from build123d import *

# Parameters (mm, degrees)
SKETCH2_W               = 70.5
SKETCH2_H               = 90
BOSS_EXTRUDE1_DEPTH     = 55.25
CUT_EXTRUDE1_DEPTH      = 91
SKETCH4_R               = 25
CUT_EXTRUDE2_DEPTH      = 45
SKETCH6_W               = 16.5
SKETCH6_H               = 50
CUT_EXTRUDE3_DEPTH      = 35.414718703
CUT_EXTRUDE3_DEPTH_BACK = 11
SKETCH7_W               = 25
SKETCH7_H               = 15
CUT_EXTRUDE4_DEPTH      = 15


with BuildPart() as part:
    # Sketch2 → Boss-Extrude1 (new body)
    with BuildSketch(Plane.XY):
        Rectangle(SKETCH2_W, SKETCH2_H)
    extrude(amount=BOSS_EXTRUDE1_DEPTH)

    # Sketch3 → Cut-Extrude1 (cut, through all)
    with BuildSketch(Plane.XZ.offset(45)):
        Polygon((28.75, 20.835281297), (35.25, 11), (35.25, 55.25), (8.75, 55.25), (8.75, 20.835281297), align=None)
    extrude(amount=-CUT_EXTRUDE1_DEPTH, mode=Mode.SUBTRACT)

    # Sketch4 → Cut-Extrude2 (cut, through all)
    with BuildSketch(Plane(origin=(8.75, 0, 0), x_dir=(0, 0, -1), z_dir=(1, 0, 0))):
        with Locations((-55.327535333, 0)):
            Circle(SKETCH4_R)
    extrude(amount=-CUT_EXTRUDE2_DEPTH, mode=Mode.SUBTRACT)

    # Sketch6 → Cut-Extrude3 (cut, two sides)
    with BuildSketch(Plane.XY.offset(20.835281297)) as cut_extrude3_sk:
        with Locations((27, 0)):
            Rectangle(SKETCH6_W, SKETCH6_H)
    extrude(amount=CUT_EXTRUDE3_DEPTH, mode=Mode.SUBTRACT)
    extrude(cut_extrude3_sk.sketch, amount=-CUT_EXTRUDE3_DEPTH_BACK, mode=Mode.SUBTRACT)

    # Sketch7 → Cut-Extrude4 (cut)
    with BuildSketch(Plane.XY.offset(55.25)):
        with Locations((-13.733691731, 26)):
            Rectangle(SKETCH7_W, SKETCH7_H)
        Polygon((-25.955312552, -17.750715844), (-0.958260941, -17.366774787), (-0.727896306, -32.365005754), (-25.724947918, -32.748946811), align=None)
    extrude(amount=-CUT_EXTRUDE4_DEPTH, mode=Mode.SUBTRACT)


solid = part.part
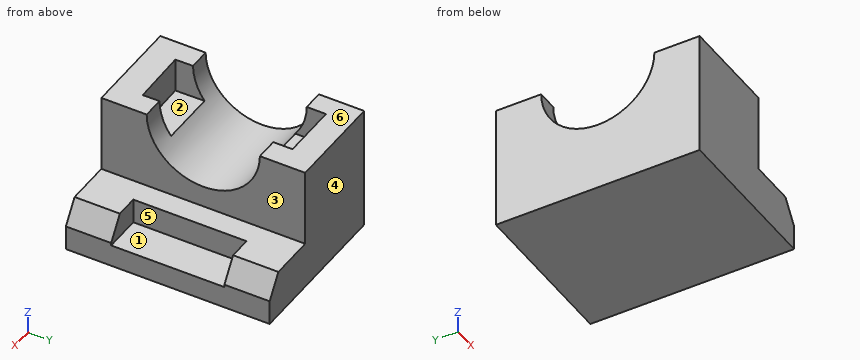
The listing builds one solid part. Answer for the finished solid, in the listing's coordinates (mm). Face numbers are marked on the shaded views. A direction names the side the tool comes from. Round coordinates to 2 decimals unless told otherwise and drop trailing zeros. Order: outer loops, then holes, each group sorted by start corner. A loop starts at its lowest first (then second) coordinate and runs counter-clockwise, first axis right, second up. Notation, with made-up numbers: (65.5, 81) -> (91.5, 81) arc R20 ccw to (91.5, 109) -> close; hole circle Ø5 at (68.25, 22). An arc over 180 degrees is marked (long way). Put each result on its own line as item: value.
Q1. Determine the mould class of the marked faces 4, 5 and 6 for opening direction Y: pulls with the +Y half, pulls with the -Y half, needs draft (parallel to the pull), parting line crosses it, or undercut.
Results list:
face 4: pulls with the +Y half
face 5: undercut
face 6: needs draft
Q2. Which of the six approach directions +Z, -Z, +X, -X, +Y, -Y give full straight-line access (tool end or side, diameter ignored) to the marked faces 1, 2 and 3?
Results list:
face 1: +Z, +X
face 2: +Z
face 3: +Z, +X, +Y, -Y
Q3. Consider line 1 along Y through (x, z) = (31, 16.5); line 2 along X through (y, z) = (17, 36); line 3 along Y through (x, z) = (-23, 35). Determine where each line is inside the solid, lowest interval first.
Results list:
line 1: -45 to -25, 25 to 45
line 2: -35.25 to 8.75
line 3: -45 to -14.55, 14.55 to 45
Q4. Section B-B, the plane y = 0 is taken. Write down the section's boundary in (x, z), and give its area (3 significant figures).
Results list:
outline: (-35.25, 0) -> (35.25, 0) -> (35.25, 9.84) -> (18.75, 9.84) -> (18.75, 20.84) -> (8.75, 20.84) -> (8.75, 30.33) -> (-35.25, 30.33) -> close
area: 1,710 mm^2
Q5. Section A-A, the plane z = 34.5 is taken. Write down the section's boundary in (x, y).
Results list:
outline: (-35.25, -45) -> (8.75, -45) -> (8.75, -13.83) -> (-35.25, -13.83) -> close; (-35.25, 13.83) -> (8.75, 13.83) -> (8.75, 45) -> (-35.25, 45) -> close
Q6. Section C-C, the plane x = 7 is taken. Write down the section's boundary in (y, z).
Results list:
outline: (-45, 0) -> (45, 0) -> (45, 55.25) -> (25, 55.25) arc R25 cw to (-25, 55.25) -> (-45, 55.25) -> close
Q7. Section D-D, the plane z = 26 is taken. Write down the section's boundary in (x, y), and give its area (3 significant figures).
Results list:
outline: (-35.25, -45) -> (8.75, -45) -> (8.75, 45) -> (-35.25, 45) -> close
area: 3,960 mm^2
Q8. Each of these flat-tipped pins is pushed along its axis until it touches: P1, Ø5, axis at x = 9.5, z = 33.5, coming from the -Y side; P2, Ø15, axis at y = 27.5, z = 48, coming from the +X side; P3, Ø13, axis at x = 24.5, y = -8.5, coming from the +Z side; P4, Ø3.5, axis at y = -8, z = 17.5, coming from the +X side. Where does it stop, or does it pass through?
Results list:
P1: y = -45
P2: x = 8.75
P3: z = 20.84
P4: x = 18.75
